Design review of the part built by this model. Coordinates are the model's own, in mm. A direction names the side the tool comes from. Give positions to 0.01 mm unless a question says otherwise; leave off trailing zeros. Write each loop counter-clockwise with the first axis right and the second up, starting at its lowest first coordinate (ties: lowest second). Pieces come first, ordered by that corner, then holes. Notation, with made-up numbers: M 29,36.5 L 57,36.5 A33 ccw 57,67.5 Z; hole C 25.5,-33.75 d5. An arc over 180 degrees is marked long. One line per item, written item: value. Start each with the question number.
```python
from build123d import *

# Parameters (mm, degrees)
CHAMFER1_SIZE = 0.762
CHAMFER2_SIZE = 2.54


with BuildPart() as part:
    # Sketch1 → Revolve1 (revolve)
    with BuildSketch(Plane.XY, mode=Mode.PRIVATE) as revolve1_sk:
        Polygon((0, 3.1115), (0, 4.7752), (20.8026, 4.7752), (20.8026, 7.62), (25.8826, 7.62), (25.8826, 4.7752), (38.8874, 4.7752), (38.8874, 7.62), (43.9674, 7.62), (43.9674, 4.7752), (64.77, 4.7752), (64.77, 3.1115), align=None)
    revolve(revolve1_sk.sketch.rotate(Axis((0, 0, 0), (1, 0, 0)), 90), axis=Axis((0, 0, 0), (1, 0, 0)))

    # Chamfer1
    chamfer1_edges = [part.edges().sort_by_distance(p)[0] for p in [
        (38.8874, 0, -7.62),
        (25.8826, 0, -7.62),
    ]]
    chamfer(chamfer1_edges, length=CHAMFER1_SIZE)

    # Chamfer2
    chamfer2_edges = [part.edges().sort_by_distance(p)[0] for p in [
        (43.9674, 0, -4.7752),
        (20.8026, 0, -4.7752),
    ]]
    chamfer(chamfer2_edges, length=CHAMFER2_SIZE)


solid = part.part
```
Q1. For P1, Ø2, axis at x = 34, y = 3.5, coming from the -Z side; P2, Ø5.5, axis at y = 0, z = 0, coming from the +X side; P3, Ø5, axis at x = 47.5, z = -3.5, coming from the +Y side; P4, Ø4, axis at x = 49, z = -0.5, coming from the +Y side, all flat-tipped, find the tip position at first contact; note any pin that passes through.
Q2. Wall thickness on line 1 (Y direction, x = 47.5, z = 0); line 2 (Y direction, x = 21, z = 0); line 3 (X direction, y = 3.75, z = -4): over which ranges is each line inside the solid? List them lowest first. Write a range as from..to.
Q3. Take a section at C-C, the plane x = 42.5. Give the boundary of the cut face in (y, z), then the cut area to 3 significant figures.
Q4. Take a section at D-D, the plane x = 49. Give the boundary of the cut face in (y, z).
Q5. The part is to be moulded in two halves that separate along X. For faces 4 (the face through (32.48, 4.66, -1.04)), 5 (the face through (0, 0.99, -3.12)), 6 (the face through (55.77, 4.66, -1.04)), say which applies: pulls with the +X half, pulls with the -X half, needs draft (parallel to the pull), parting line crosses it, or undercut.
Q6. Machinability: for faces 1 (the face through (22.992, -7.555, -0.992)), 2 (the face through (25.883, 1, -5)), 3 (the face through (9.26, 4.66, -1.04)), which of the approach directions +Z, -Z, +X, -X, +Y, -Y give a long, thin tool a straight path to every point of the face, cutting with its end or side? Answer none if there is none.
Results list:
1. P1: stops at z = -4.07
1. P2: passes through
1. P3: stops at y = 5.54
1. P4: stops at y = 4.78
2. line 1: y = -4.78..-3.11, 3.11..4.78
2. line 2: y = -7.62..-3.11, 3.11..7.62
2. line 3: x = 18.97..25.88, 38.89..45.8
3. outline: C 0,0 d15.24; hole C 0,0 d6.22
3. area: 152 mm^2
4. outline: C 0,0 d9.55; hole C 0,0 d6.22
5. face 4: undercut
5. face 5: pulls with the -X half
5. face 6: needs draft
6. face 1: +X, -X
6. face 2: none
6. face 3: -X
